Part model, mm, in its own coordinate system. A direction names the side the tool comes from. Round coordinates to 2 decimals unless told otherwise and drop trailing zeros. Write each loop counter-clockwise with the first axis right and the second up, starting at its lowest first coordinate (ties: lowest second). Pieces come first, ordered by that corner, then holes.
1) Drill centre lines: L1, parallel to Y at x = 39.5, z = 16.5; L2, parallel to X at y = 9.5, z = 30; L3, parallel to X at y = 35.5, z = 16. Where is each one in solid material? Low to high.
2) Which spindle directions (+Z, -Z, +X, -X, +Y, -Y) get a long thin tool onto all of the face, cutting with end or side? Do faces 1 (the flat face through (85, 25, 15)), 2 (the flat face through (42, 48, 30)). Say none if no direction does.
3) Saw through at B-B on x = 17. Write the cut outline in (y, z), and give its area (3 significant figures).
4) Saw through at C-C on y = 14.5. Write the cut outline in (x, z).
5) Flat gauge pin, fed straight in: pin 1 (8 mm diameter, centred on x = 25.5, y = 40.5, fed in from +Z). Where does the tip first touch, or does it go through?
6) Saw through at A-A on z = 14.5. Write the cut outline in (x, y), and give its area (3 significant figures).
```python
from build123d import *

# Parameters (mm, degrees)
SKICA1_W                = 85
SKICA1_H                = 50
P_IDAT_VYSUNUT_M1_DEPTH = 3
SKICA1_5_W              = 85
SKICA1_5_H              = 50
SKICA1_5_W_2            = 81
SKICA1_5_H_2            = 46
P_IDAT_VYSUNUT_M2_DEPTH = 31
SKICA1_6_W              = 81
SKICA1_6_H              = 46
SKICA1_6_W_2            = 77
SKICA1_6_H_2            = 42
P_IDAT_VYSUNUT_M3_DEPTH = 29


with BuildPart() as part:
    # Skica1 → Přidat vysunutím1 (new body)
    with BuildSketch(Plane.XY):
        with Locations((42.5, 25)):
            Rectangle(SKICA1_W, SKICA1_H)
    extrude(amount=P_IDAT_VYSUNUT_M1_DEPTH)

    # Skica1<5> → Přidat vysunutím2 (add)
    with BuildSketch(Plane.XY):
        with Locations((42.5, 25)):
            Rectangle(SKICA1_5_W, SKICA1_5_H)
        with Locations((42.5, 25)):
            Rectangle(SKICA1_5_W_2, SKICA1_5_H_2, mode=Mode.SUBTRACT)
    extrude(amount=P_IDAT_VYSUNUT_M2_DEPTH)

    # Skica1<6> → Přidat vysunutím3 (add)
    with BuildSketch(Plane.XY):
        with Locations((42.5, 25)):
            Rectangle(SKICA1_6_W, SKICA1_6_H)
        with Locations((42.5, 25)):
            Rectangle(SKICA1_6_W_2, SKICA1_6_H_2, mode=Mode.SUBTRACT)
    extrude(amount=P_IDAT_VYSUNUT_M3_DEPTH)


solid = part.part
```
Completed:
1. L1: y = 0 to 4, 46 to 50
1. L2: x = 0 to 2, 83 to 85
1. L3: x = 0 to 4, 81 to 85
2. face 1: +Z, -Z, +X, +Y, -Y
2. face 2: +Z
3. outline: (0, 0) - (50, 0) - (50, 31) - (48, 31) - (48, 29) - (46, 29) - (46, 3) - (4, 3) - (4, 29) - (2, 29) - (2, 31) - (0, 31) - close
3. area: 366 mm2
4. outline: (0, 0) - (85, 0) - (85, 31) - (83, 31) - (83, 29) - (81, 29) - (81, 3) - (4, 3) - (4, 29) - (2, 29) - (2, 31) - (0, 31) - close
5. pin 1: stops at z = 3
6. outline: (0, 0) - (85, 0) - (85, 50) - (0, 50) - close; hole (4, 4) - (81, 4) - (81, 46) - (4, 46) - close
6. area: 1,020 mm2
